Verification items for this drawing (mm, ordinates from the low corner). Round coordinates to 2 decimals unless told otherwise and drop trailing zeros. Write each loop counter-clockwise with the first axis right and the second up, starting at its lowest first coordinate (ties: lowest second). Pieces come first, ordered by that corner, then holes.
Item 1: Scan lines: probe 1 along Z at (x, y) = (43, 7); probe 2 along Y at (x, z) = (16, 1.75); probe 3 along Y at (x, z) = (28, 13.5). Record each from-to range of solid material in increasing order.
Item 2: Cross-section at D-D (y = 3.75). Enter the section's corners in (x, z).
Item 3: Cross-section at A-A (z = 10.5). Enter the section's corners in (x, y).
Item 4: Cross-section at C-C (x = 38). Enter the section's corners in (y, z), then the cut area to 3 significant figures.
Item 5: Depth check by flat-ended pin: P1, Ø3, axis at x = 30, z = 12, coming from the +Y side; P2, Ø1.5, axis at x = 45.5, z = 2, coming from the +Y side; P3, Ø1.5, axis at x = 30.5, z = 9, coming from the +Y side. Enter the tip coordinate at first touch or a pass-through.
Item 6: Cross-section at B-B (y = 9.75). Enter the section's corners in (x, z).
Item 7: Draft check along Y on the marked faces 1 and 2. Enter one of: pulls with the +Y half, pulls with the -Y half, needs draft (parallel to the pull), parting line crosses it, or undercut.
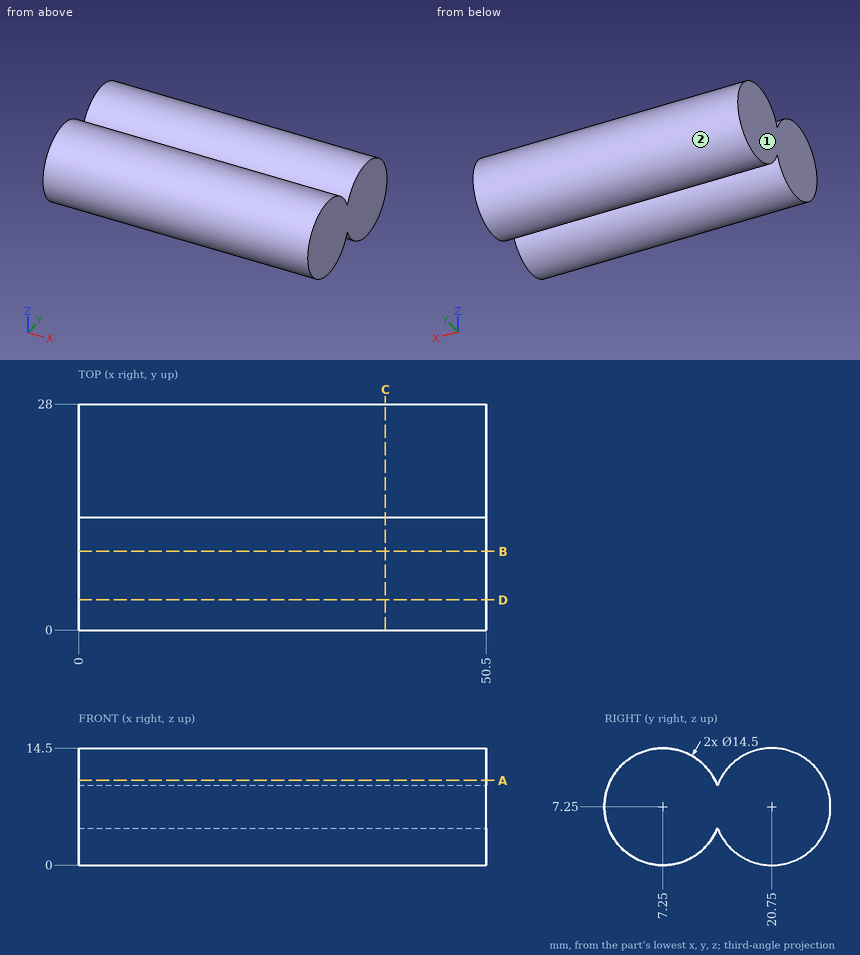
Resolved:
1. probe 1: z = 0 to 14.5
1. probe 2: y = 2.53 to 11.97, 16.03 to 25.47
1. probe 3: y = 3.58 to 10.92, 17.08 to 24.42
2. outline: (0, 0.9) - (50.5, 0.9) - (50.5, 13.6) - (0, 13.6) - close
3. outline: (0, 0.77) - (50.5, 0.77) - (50.5, 13.73) - (0, 13.73) - close; (0, 14.27) - (50.5, 14.27) - (50.5, 27.23) - (0, 27.23) - close
4. outline: (14, 4.6) arc R7.25 ccw (long way) to (14, 9.9) arc R7.25 ccw (long way) to start
4. area: 327 mm2
5. P1: stops at y = 27.23
5. P2: stops at y = 26.43
5. P3: stops at y = 27.93
6. outline: (0, 0.44) - (50.5, 0.44) - (50.5, 14.06) - (0, 14.06) - close
7. face 1: needs draft
7. face 2: undercut
